Geometry: final body of the model. Coordinates: model frame, mm. Face numbers are marked on the shaded views. Coordinates: 2 decimals unless noted, no trailing zeros. Loops run counter-clockwise (first coordinate to the right, second up) from the corner with the lowest first, then second, coordinate; pieces in that order, holes last. Notation, with made-up numbers: (-7, -17.5) -> (8, -17.5) arc R22 cw to (8, 11.5) -> close; hole circle Ø5 at (79, 15). An arc over 180 degrees is marked (long way). One line per item, written item: value. Start each with the question number.
Item 1: Section query B-B on z = 28.5. Return loops of the section in (x, y).
Item 2: Section query A-A on z = 53.5. Return loops of the section in (x, y), then the cut area to 3 significant figures.
Item 3: Mould query, pull axis X, two halves, no side actions, for the marked faces 1, 2 and 3. Classes: +X half, -X half, draft (parallel to the pull), parting line (faces both ways), or undercut.
Item 4: Ray query, probe 1 along X at (y, z) = (0, 3.5); probe 2 along X at (y, z) = (-6.5, 27). Return the intervals inside material, ascending. Write a range as from..to.
Item 5: Contact query for flat-ended pins moving along their axis: pin 1 Ø10 at (x, z) = (-2.5, 23.5) entering from -Y; pin 2 Ø1.5 at (y, z) = (2.5, 52) entering from +X; pin 3 Ø2 at (x, z) = (1.5, 47.5) entering from +Y; pin 4 Ø5 at (x, y) = (0, 0) entering from -Z. Output: stop coordinate, or through.
from build123d import *

# Parameters (mm, degrees)
SKETCH_1_R               = 10
EXTRUDE_1_DEPTH          = 64
CHAMFER_1_SIZE           = 1
CUT_EXTRUDE_1_DEPTH      = 66.543878433
CUT_EXTRUDE_1_DEPTH_BACK = 66.543878433
F_8_0MM_1_D              = 8
F_8_0MM_1_DEPTH          = 9.190598923
F_8_0MM_1_CSINK_D        = 12
F_8_0MM_1_CSINK_ANGLE    = 90
F_8_0MM_1_TIP            = 2.309401077


with BuildPart() as part:
    # 草图1 → 凸台-拉伸1 (new body)
    with BuildSketch(Plane.XY):
        Circle(SKETCH_1_R)
    extrude(amount=EXTRUDE_1_DEPTH)

    # 倒角1
    chamfer_1_edges = [part.edges().sort_by_distance(p)[0] for p in [
        (-10, 0, 64),
    ]]
    chamfer(chamfer_1_edges, length=CHAMFER_1_SIZE)

    # 草图2 → 切除-拉伸1 (cut, two sides: drawn at the far end of the back side and taken through both)
    with BuildSketch(Plane(origin=(0, 0, 0), x_dir=(0, 0, -1), z_dir=(1, 0, 0)).offset(-CUT_EXTRUDE_1_DEPTH_BACK)):
        Polygon((-200.698918074, -29.684080093), (-64, -0.627828084), (-14, 10), (122.698918074, 39.05625201), (64.586414054, 312.454088158), (-258.811422094, 243.713756055), align=None)
    extrude(amount=CUT_EXTRUDE_1_DEPTH + CUT_EXTRUDE_1_DEPTH_BACK, mode=Mode.SUBTRACT)

    # Ø8.0mm 暗销孔1
    with Locations(Plane(origin=(0, 0, 0), x_dir=(-1, 0, 0), z_dir=(0, 0, -1))):
        with Locations((0, 0)):
            CounterSinkHole(F_8_0MM_1_D / 2, F_8_0MM_1_CSINK_D / 2, depth=F_8_0MM_1_DEPTH, counter_sink_angle=F_8_0MM_1_CSINK_ANGLE)
            with Locations((0, 0, -(F_8_0MM_1_DEPTH + F_8_0MM_1_TIP / 2))):  # 120° drill point
                Cone(0, F_8_0MM_1_D / 2, F_8_0MM_1_TIP, mode=Mode.SUBTRACT)


solid = part.part
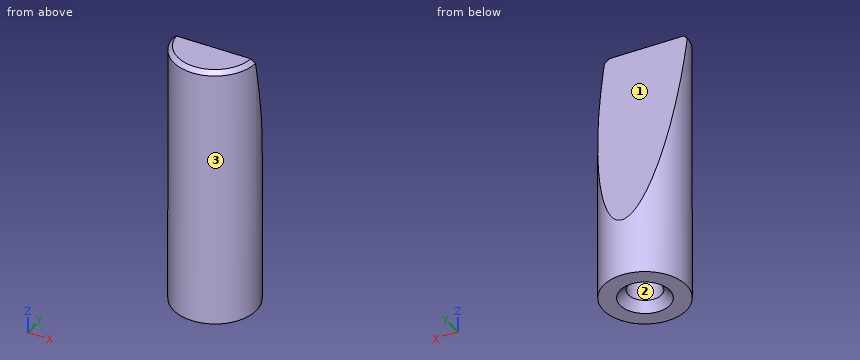
Reply:
1. outline: (-7.22, 6.92) arc R10 ccw (long way) to (7.22, 6.92) -> close
2. outline: (-9.87, 1.6) arc R10 ccw (long way) to (9.87, 1.6) -> close
2. area: 189 mm²
3. face 1: draft
3. face 2: undercut
3. face 3: parting line
4. probe 1: x = -10..-4, 4..10
4. probe 2: x = -7.6..7.6
5. pin 1: stops at y = -10
5. pin 2: stops at x = 9.85
5. pin 3: stops at y = 3.09
5. pin 4: stops at z = 10.06
